Input: part model. Units: mm. Frame: model coordinates. Face numbers are marked on the shaded views. Give positions to 0.01 mm unless a question says otherwise; leave off trailing zeros. Loops run counter-clockwise (first coordinate to the right, second up) from the corner with the lowest first, then second, coordinate; pieces in that order, holes last. Notation, with made-up numbers: (36, 84) -> (45, 84) arc R19 ccw to (45, 116) -> close; hole circle Ø8 at (89, 64). An arc over 180 degrees is marked (long way). Answer as a JSON object with one key per item and string values.
Autodesk Inventor part; units mm, degrees
ref_plane "YZ Plane" through (0, 0, 0) normal (1, 0, 0) x (0, 1, 0)
ref_plane "XZ Plane" through (0, 0, 0) normal (0, 1, 0) x (-1, 0, 0)
ref_plane "XY Plane" through (0, 0, 0) normal (0, 0, 1) x (1, 0, 0)
sketch "Sketch1" plane through (0, 0, 0) normal (0, 0, 1) x (1, 0, 0)
  line L0 (3, -6) -> (-3, -6)
  line L1 (3, 21) -> (3, -6)
  line L2 (-3, 21) -> (3, 21)
  line L3 (-3, -6) -> (-3, 21)
  circle A0 centre (15.8383, 17.8821) radius 1.5
  line L4 (18.8902, -6) -> (18.8902, 21)
  line L5 (13, 21) -> (18.8902, 21)
  line L6 (13, -6) -> (13, 21)
  line L7 (18.8902, -6) -> (13, -6)
  circle A1 centre (0.0519, 34.1179) radius 1.5
  line L8 (3, 46) -> (3, 31)
  line L9 (-3, 46) -> (3, 46)
  line L10 (-3, 31) -> (-3, 46)
  line L11 (3, 31) -> (-3, 31)
  line L12 (18.8902, 14.8821) -> (-3, 14.8821)
  line L13 (-3, 14.8821) -> (-3, 37.1179)
  line L14 (-3, 37.1179) -> (13, 37.1179)
  line L15 (18.8902, 21) -> (18.8902, 14.8821)
  line L16 (18.8902, 21) -> (13, 37.1179)
  point P0 (0, 0)
  dimension "d0" = 3
  dimension "d1" = 3
extrude "Extrusion1" add sketch "Sketch1" along normal blind 1.5 contours L12 L3 L2 L1 | L1 L2 L13 L11 L8 L14 L16 L5 L6 L12 | L6 L5 L4 L12 | L10 L14 L8 L11
properties part number "top_plate"
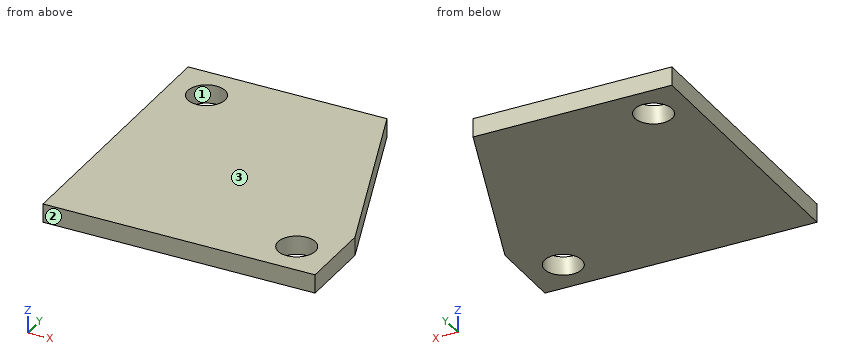
Q1. Section C-C, the plane z = 1.15. Return the cut outline in (x, y).
Evaluation:
{"outline": "(-3, 14.88) -> (18.89, 14.88) -> (18.89, 21) -> (13, 37.12) -> (-3, 37.12) -> close; hole circle Ø3 at (0.05, 34.12); hole circle Ø3 at (15.84, 17.88)"}
Q2. Draft query along Y for the marked faces 1, 2 and 3. Return one class per face: +Y half, -Y half, draft (parallel to the pull), parting line (faces both ways), or undercut.
Evaluation:
{"face 1": "undercut", "face 2": "-Y half", "face 3": "draft"}
Q3. Pin query (flat end, axial travel): pin 1 (2.5 mm diameter, centred on x = 0.05, y = 34.12, fed in from -Z). Return the tip coordinate at first contact, or that it passes through.
Evaluation:
{"pin 1": "passes through"}
Q4. Section B-B, the plane y = 17.25. Return the cut outline in (x, z), then the cut area to 3 significant figures.
Evaluation:
{"outline": "(-3, 0) -> (14.48, 0) -> (14.48, 1.5) -> (-3, 1.5) -> close; (17.2, 0) -> (18.89, 0) -> (18.89, 1.5) -> (17.2, 1.5) -> close", "area": "28.8 mm2"}
Q5. Section A-A, the plane x = -0.25. Return the cut outline in (y, z).
Evaluation:
{"outline": "(14.88, 0) -> (32.65, 0) -> (32.65, 1.5) -> (14.88, 1.5) -> close; (35.59, 0) -> (37.12, 0) -> (37.12, 1.5) -> (35.59, 1.5) -> close"}
Q6. Ray query, line 1 along Y through (x, z) = (0, 0.85); line 2 along X through (y, z) = (34.5, 0.95); line 3 along X through (y, z) = (33, 1.35). Return the intervals inside material, ascending.
Evaluation:
{"line 1": "y = 14.88 to 32.62, 35.62 to 37.12", "line 2": "x = -3 to -1.4, 1.5 to 13.96", "line 3": "x = -3 to -0.95, 1.05 to 14.5"}
Q7. Section D-D, the plane y = 31.75. Return the cut outline in (x, z).
Evaluation:
{"outline": "(-3, 0) -> (14.96, 0) -> (14.96, 1.5) -> (-3, 1.5) -> close"}
